Drawing for the job (mm, zero at the part's lowest x, y, z). A direction names the side the tool comes from. Give positions to 0.01 mm unless a question says otherwise; leave off trailing zeros. Order: outer loops, then holes, each group sorted by start corner. A loop starts at its lowest first (then second) coordinate and runs counter-clockwise, first axis right, second up. Notation, with made-up numbers: (66, -2) - (102, -2) arc R21 ccw to (102, 30) - close; hole circle Ø11 at (4.5, 66). An arc over 180 degrees is marked (long way). Use a Markdown table: item, result.
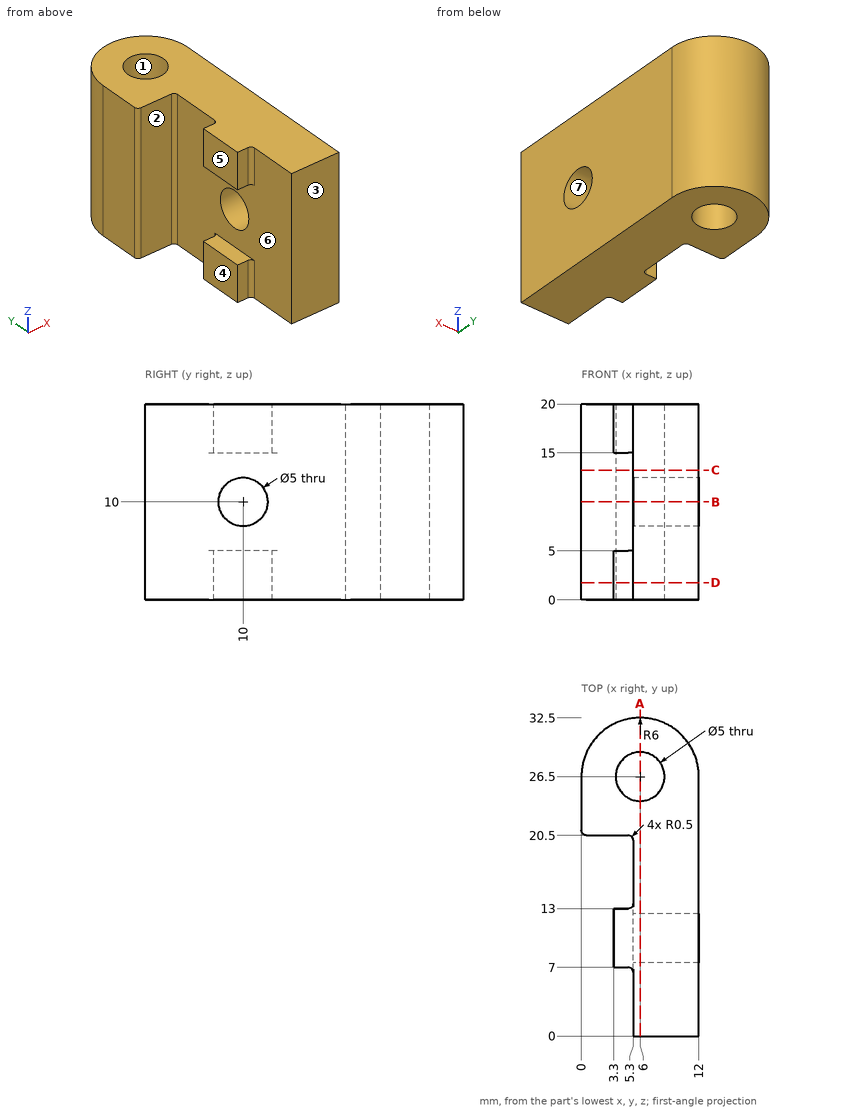
1) Slice it at D-D (z = 1.75). Write the cut outline in (x, y), and give its area (3 significant figures).
Computed:
| item | result |
|---|---|
| outline | (0, 21) arc R0.5 ccw to (0.5, 20.5) - (4.8, 20.5) arc R0.5 cw to (5.3, 20) - (5.3, 13.5) arc R0.5 cw to (4.8, 13) - (3.3, 13) - (3.3, 7) - (4.8, 7) arc R0.5 cw to (5.3, 6.5) - (5.3, 0) - (12, 0) - (12, 26.5) arc R6 ccw to (0, 26.5) - close; hole circle Ø5 at (6, 26.5) |
| area | 258 mm² |
2) Tool access for the marked faces 5, 6 and 7: list every direction of +Z, -Z, +X, -X, +Y, -Y with a clear straight run to the whole face (end or side of a thin tool).
Computed:
| item | result |
|---|---|
| face 5 | +Z, -Z, -X, -Y |
| face 6 | -X |
| face 7 | +X, -X |
3) Wall check: line 1 (Y direction, x = 6, z = 6.5); line 2 (Y direction, x = 6, z = 9.5); line 3 (X direction, y = 6.5, z = 16.5). Give the ranges that are in metal, low to high. Write a range as from..to.
Computed:
| item | result |
|---|---|
| line 1 | y = 0..24, 29..32.5 |
| line 2 | y = 0..7.55, 12.45..24, 29..32.5 |
| line 3 | x = 5.3..12 |
4) Two-plate mould, pull along Y, no slides. Class the marked faces 1, 2, 3 and 4: +Y half, -Y half, draft (parallel to the pull), parting line (faces both ways), or undercut.
Computed:
| item | result |
|---|---|
| face 1 | undercut |
| face 2 | undercut |
| face 3 | -Y half |
| face 4 | draft |
5) Slice it at B-B (z = 10). Write the cut outline in (x, y).
Computed:
| item | result |
|---|---|
| outline | (0, 21) arc R0.5 ccw to (0.5, 20.5) - (4.8, 20.5) arc R0.5 cw to (5.3, 20) - (5.3, 12.5) - (12, 12.5) - (12, 26.5) arc R6 ccw to (0, 26.5) - close; (5.3, 0) - (12, 0) - (12, 7.5) - (5.3, 7.5) - close; hole circle Ø5 at (6, 26.5) |
6) Slice it at C-C (z = 13.25). Write the cut outline in (x, y), and give its area (3 significant figures).
Computed:
| item | result |
|---|---|
| outline | (0, 21) arc R0.5 ccw to (0.5, 20.5) - (4.8, 20.5) arc R0.5 cw to (5.3, 20) - (5.3, 0) - (12, 0) - (12, 26.5) arc R6 ccw to (0, 26.5) - close; hole circle Ø5 at (6, 26.5) |
| area | 246 mm² |
7) Slice it at A-A (x = 6). Write the cut outline in (y, z).
Computed:
| item | result |
|---|---|
| outline | (0, 0) - (24, 0) - (24, 20) - (0, 20) - close; (29, 0) - (32.5, 0) - (32.5, 20) - (29, 20) - close; hole circle Ø5 at (10, 10) |
8) Pin check, flat tips, straight feed: P1, Ø1.2, axis at x = 4, z = 18, coming from the -Y side; P2, Ø1.5, axis at x = 6.5, y = 27.5, coming from the -Z side; P3, Ø2, axis at x = 2, z = 7, coming from the -Y side; P4, Ø1.7, axis at x = 4, z = 18, coming from the +Y side. Stop position of each tip, or through.
Computed:
| item | result |
|---|---|
| P1 | stops at y = 7 |
| P2 | passes through |
| P3 | stops at y = 20.5 |
| P4 | stops at y = 32.39 |
